```python
from build123d import *

# Parameters (mm, degrees)
SKETCH1_R           = 12.5
BOSS_EXTRUDE1_DEPTH = 47
SKETCH2_W           = 35
SKETCH2_H           = 35
BOSS_EXTRUDE2_DEPTH = 36
FILLET1_R           = 2


with BuildPart() as part:
    # Sketch1 → Boss-Extrude1 (new body)
    with BuildSketch(Plane(origin=(0, 0, 0), x_dir=(1, 0, 0), z_dir=(0, 1, 0))):
        with Locations(Location((0, 0, 0), (0, 0, 270))):
            Circle(SKETCH1_R)
    extrude(amount=BOSS_EXTRUDE1_DEPTH)

    # Sketch2 → Boss-Extrude2 (add)
    with BuildSketch(Plane(origin=(0, 47, 0), x_dir=(1, 0, 0), z_dir=(0, 1, 0))):
        Rectangle(SKETCH2_W, SKETCH2_H)
    extrude(amount=BOSS_EXTRUDE2_DEPTH)

    # Fillet1
    fillet1_edges = [part.edges().sort_by_distance(p)[0] for p in [
        (0, 0, -12.5),
        (-17.5, 83, 0),
        (-17.5, 65, -17.5),
        (0, 47, 17.5),
        (-17.5, 65, 17.5),
        (17.5, 47, 0),
        (17.5, 65, 17.5),
        (0, 83, -17.5),
        (17.5, 65, -17.5),
        (0, 83, 17.5),
        (17.5, 83, 0),
        (-17.5, 47, 0),
        (0, 47, -17.5),
    ]]
    fillet(fillet1_edges, radius=FILLET1_R)


solid = part.part
```
Geometry: final body of the model. Coordinates: model frame, mm. A direction names the side the tool comes from. Coordinates: 2 decimals unless noted, no trailing zeros. Loops run counter-clockwise (first coordinate to the right, second up) from the corner with the lowest first, then second, coordinate; pieces in that order, holes last. Notation, with made-up numbers: (76.5, 84) -> (131.5, 84) arc R15 cw to (131.5, 112) -> close; hole circle Ø1 at (38.25, -40). An arc over 180 degrees is marked (long way). Use a Markdown table: item, result. Add a question column.
(1) Section query C-C, the plane y = 30.5. Return loops of the section in (x, z), plus the area to 3 significant figures.
(2) Line query: line 1 along Y through (x, z) = (13.5, -2.5); line 2 along Z through (x, y) = (-0.5, 13); line 3 along Y through (x, z) = (-10, -6). Output: solid intervals per line, ascending.
(3) Section query A-A, the plane z = 0. Return loops of the section in (x, y).
(4) Access query for faces 1 (the flat face through (0, 83, 0)), 2 (the flat face through (-7, 47, -11)). Directions: +Z, -Z, +X, -X, +Y, -Y. A direction counts if a zero-diameter tool reaches every point of the face in a straight line with its end or side. Return the directions, or none.
(5) Pin query (flat end, axial travel): pin 1 Ø10 at (x, y) = (10.5, 42.5) entering from -Z; pin 2 Ø5 at (y, z) = (19.5, -10.5) entering from -X; pin 3 Ø12 at (y, z) = (31.5, 1.5) entering from -X. Return the tip coordinate at first contact, or that it passes through.
(6) Section query B-B, the plane x = 0. Return loops of the section in (y, z).
Answer:
| question | item | result |
|---|---|---|
| 1 | outline | circle Ø25 at (0, 0) |
| 1 | area | 491 mm^2 |
| 2 | line 1 | y = 47 to 83 |
| 2 | line 2 | z = -12.49 to 12.49 |
| 2 | line 3 | y = 0.37 to 83 |
| 3 | outline | (-17.5, 49) arc R2 ccw to (-15.5, 47) -> (-12.5, 47) -> (-12.5, 2) arc R2 ccw to (-10.5, 0) -> (10.5, 0) arc R2 ccw to (12.5, 2) -> (12.5, 47) -> (15.5, 47) arc R2 ccw to (17.5, 49) -> (17.5, 81) arc R2 ccw to (15.5, 83) -> (-15.5, 83) arc R2 ccw to (-17.5, 81) -> close |
| 4 | face 1 | +Z, -Z, +X, -X, +Y |
| 4 | face 2 | -Y |
| 5 | pin 1 | stops at z = -16.82 |
| 5 | pin 2 | stops at x = -9.6 |
| 5 | pin 3 | stops at x = -12.5 |
| 6 | outline | (0, -10.5) arc R2 ccw to (2, -12.5) -> (47, -12.5) -> (47, -15.5) arc R2 ccw to (49, -17.5) -> (81, -17.5) arc R2 ccw to (83, -15.5) -> (83, 15.5) arc R2 ccw to (81, 17.5) -> (49, 17.5) arc R2 ccw to (47, 15.5) -> (47, 12.5) -> (2, 12.5) arc R2 ccw to (0, 10.5) -> close |
